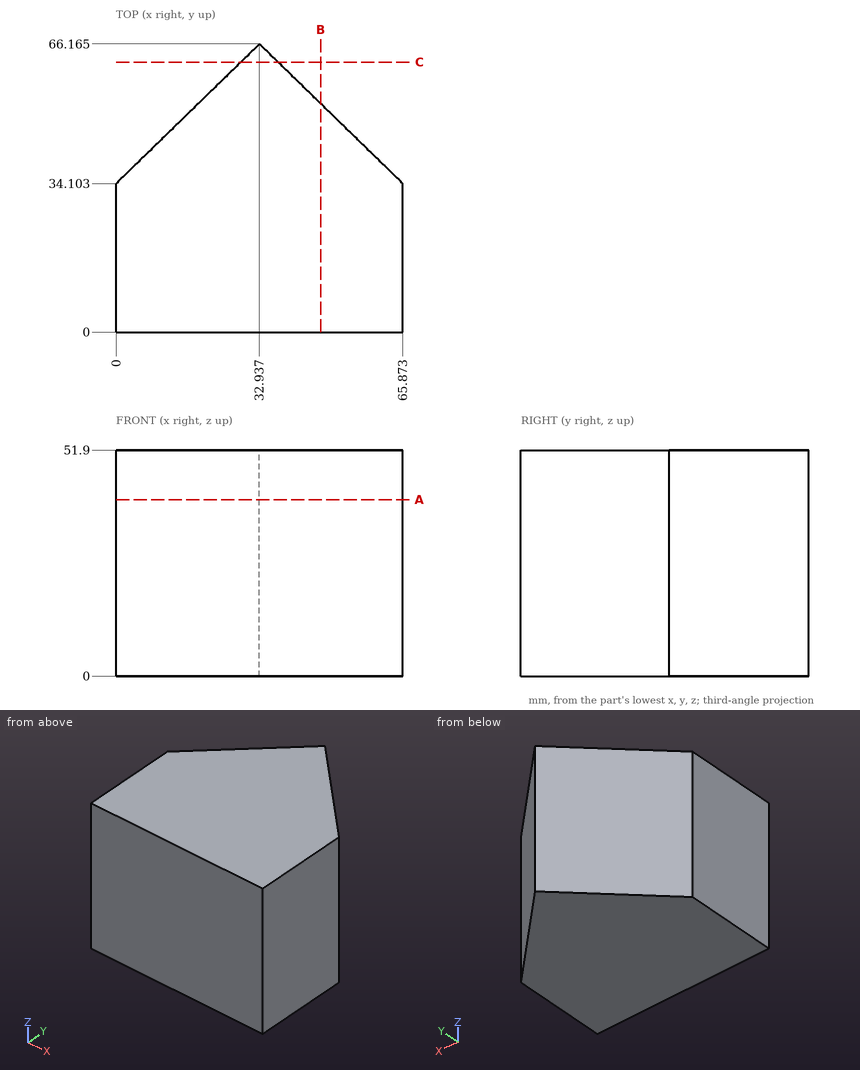
Part print with two shaded views. Sizes in mm from the minimum x, y, z corner. Coordinates: 2 decimals unless noted, no trailing zeros. Order: outer loops, then holes, each group sorted by start corner. A loop starts at its lowest first (then second) coordinate and runs counter-clockwise, first axis right, second up. Notation, with made-up numbers: (82, 60) - (126, 60) arc R32 cw to (126, 94) - close; hole circle Ø3 at (61, 54.25). An arc over 180 degrees is marked (long way). Write item = value, one per line. Start each with the question number.
1) Wall check: line 1 along Y through (x, z) = (36, 31) (1 decimal); line 2 along Y through (x, z) = (8, 28); line 3 along X through (y, z) = (59, 19) (1 decimal). Give the ranges that are in metal, low to high. Write a range as from..to.
2) Saw through at B-B on x = 47. Write the cut outline in (y, z) (1 decimal), then the cut area to 3 significant figures.
3) Flat gauge pins, fed straight in: pin 1 Ø12 at (x, z) = (49, 19.5) entering from -Y; pin 2 Ø5 at (x, z) = (32, 15.5) entering from +Y (1 decimal); pin 3 Ø5 at (y, z) = (49, 16.5) entering from -X (1 decimal); pin 4 Ø5 at (y, z) = (39, 22.5) entering from +X. Where does each tip first touch, or does it go through?
4) Saw through at C-C on y = 62. Write the cut outline in (x, z) (1 decimal).
5) Saw through at A-A on z = 40.5. Write the cut outline in (x, y) (1 decimal), then the cut area to 3 significant figures.
From the geometry:
q1.line_1 = 0..63.2
q1.line_2 = 0..41.89
q1.line_3 = 25.6..40.3
q2.outline = (0, 0) - (52.5, 0) - (52.5, 51.9) - (0, 51.9) - close
q2.area = 2,720 mm^2
q3.pin_1 = 0
q3.pin_2 = 66.2
q3.pin_3 = 12.7
q3.pin_4 = 63.41
q4.outline = (28.7, 0) - (37.2, 0) - (37.2, 51.9) - (28.7, 51.9) - close
q5.outline = (0, 0) - (65.9, 0) - (65.9, 34.1) - (32.9, 66.2) - (0, 34.1) - close
q5.area = 3,300 mm^2
